Read the model definition and answer for the solid it produces. Units are mm, in the model's axes. Face numbers are marked on the shaded views. A direction names the side the tool comes from. Coordinates: 2 decimals unless noted, no trailing zeros. Loops run counter-clockwise (first coordinate to the right, second up) from the corner with the lowest first, then second, coordinate; pieces in that order, holes last.
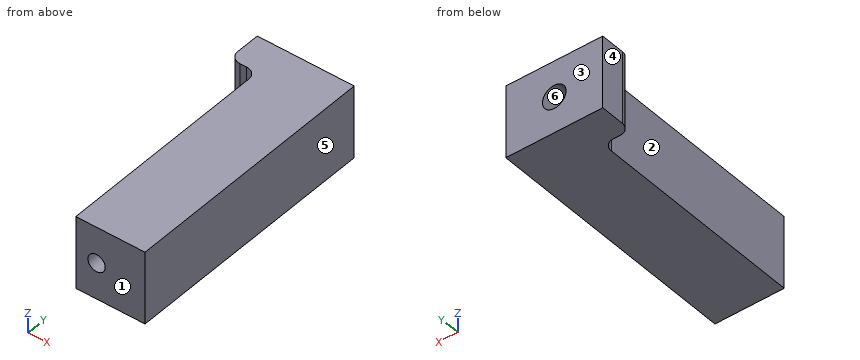
from build123d import *

# Parameters (mm, degrees)
SKETCH_1_W             = 28
SKETCH_1_H             = 21
EXTRUDE_1_DEPTH        = 75
SKETCH_6_W             = 8
SKETCH_6_H             = 65
CUT_EXTRUDE_1_DEPTH    = 22
FILLET_3_R             = 3
HOLE_WIZARD_M6_1_D     = 5
HOLE_WIZARD_M6_1_DEPTH = 19.75
HOLE_WIZARD_M6_1_TIP   = 1.502151548


with BuildPart() as part:
    # 草图1 → 凸台-拉伸1 (new body)
    with BuildSketch(Plane(origin=(0, 0, 0), x_dir=(1, 0, 0), z_dir=(0, 1, 0))):
        Rectangle(SKETCH_1_W, SKETCH_1_H)
    extrude(amount=EXTRUDE_1_DEPTH)

    # 草图5 → M8 螺纹孔1 (revolve, cut)
    with BuildSketch(Plane(origin=(0, 75, 0), x_dir=(0, 0, 1), z_dir=(1, 0, 0))):
        Polygon((0, 0), (0, 21.792926105), (3.4, 19.75), (3.4, 0), align=None)
    revolve(axis=Axis((0, 81.35, 0), (0, -1, 0)), mode=Mode.SUBTRACT)

    # 草图6 → 切除-拉伸1 (cut, through all)
    with BuildSketch(Plane.XY.offset(10.5)):
        with Locations((-10, 32.5)):
            Rectangle(SKETCH_6_W, SKETCH_6_H)
    extrude(amount=-CUT_EXTRUDE_1_DEPTH, mode=Mode.SUBTRACT)

    # 圆角3
    fillet_3_edges = [part.edges().sort_by_distance(p)[0] for p in [
        (-14, 65, 0),
        (-6, 65, 0),
    ]]
    fillet(fillet_3_edges, radius=FILLET_3_R)

    # M6 螺纹孔1
    with Locations(Plane(origin=(0, 0, 0), x_dir=(0, 0, -1), z_dir=(0, -1, 0))):
        with Locations((0, 0)):
            Hole(HOLE_WIZARD_M6_1_D / 2, depth=HOLE_WIZARD_M6_1_DEPTH)
            with Locations((0, 0, -(HOLE_WIZARD_M6_1_DEPTH + HOLE_WIZARD_M6_1_TIP / 2))):  # 118° drill point
                Cone(0, HOLE_WIZARD_M6_1_D / 2, HOLE_WIZARD_M6_1_TIP, mode=Mode.SUBTRACT)


solid = part.part
Item 1: A cutting plane is placed at B-B on z = -7.75. Determine the outline of the cut face in (x, y), then the cut area to 3 significant figures.
Numbers:
outline: (-14, 68) arc R3 ccw to (-11, 65) - (-9, 65) arc R3 cw to (-6, 62) - (-6, 0) - (14, 0) - (14, 75) - (-14, 75) - close
area: 1,580 mm2
Item 2: A cutting plane is placed at C-C on x = -10. Determine the outline of the cut face in (y, z).
Numbers:
outline: (65, -10.5) - (75, -10.5) - (75, 10.5) - (65, 10.5) - close
Item 3: Determine the mould class of the marked faces 3, 4, 5 and 6 for opening direction X: released by +X, released by -X, zero draft, split by the parting line, or undercut.
Numbers:
face 3: zero draft
face 4: released by -X
face 5: released by +X
face 6: undercut
Item 4: Which of the six approach directions +Z, -Z, +X, -X, +Y, -Y give full straight-line access (tool end or side, diameter ignored) to the marked faces 1 and 2?
Numbers:
face 1: +Z, -Z, +X, -X, -Y
face 2: +Z, -Z, -X, -Y
Item 5: Given pin 1 (5 mm diameter, centred on y = 17, z = -7, fed in from -X); pin 2 (8 mm diameter, centred on x = 0, z = 0, fed in from +Y); pin 3 (3 mm diameter, centred on x = 0, z = 0, fed in from +Y); pin 4 (1.6 mm diameter, centred on x = -10, z = 2.5, fed in from -Y), each flat-ended and moving along its own axis, determine where each tip first touches the part or whether it passes through.
Numbers:
pin 1: stops at x = -6
pin 2: stops at y = 75
pin 3: stops at y = 54.11
pin 4: stops at y = 65
Item 6: A cutting plane is placed at A-A on y = 12. Determine the outline of the cut face in (x, z), then the cut area to 3 significant figures.
Numbers:
outline: (-6, -10.5) - (14, -10.5) - (14, 10.5) - (-6, 10.5) - close; hole circle Ø5 at (0, 0)
area: 400 mm2
Item 7: A cutting plane is placed at D-D on y = 26. Determine the outline of the cut face in (x, z), then the cut area to 3 significant figures.
Numbers:
outline: (-6, -10.5) - (14, -10.5) - (14, 10.5) - (-6, 10.5) - close
area: 420 mm2
Item 8: Find the intervals of material crossed by line 1 along X through (y, z) = (62, 0); line 2 along Z through (x, y) = (0, 6.25); line 3 along Z through (x, y) = (0, 63.5), in increasing order.
Numbers:
line 1: x = -6 to -3.4, 3.4 to 14
line 2: z = -10.5 to -2.5, 2.5 to 10.5
line 3: z = -10.5 to -3.4, 3.4 to 10.5
